Input: dimensioned drawing with shaded views. Units: mm. Origin: part minimum x, y, z. Give positions to 0.01 mm unless a question says otherwise; leave off trailing zeros. Order: outer loops, then holes, each group sorted by start corner. A loop starts at its lowest first (then second) coordinate and runs counter-clockwise, first axis right, second up.
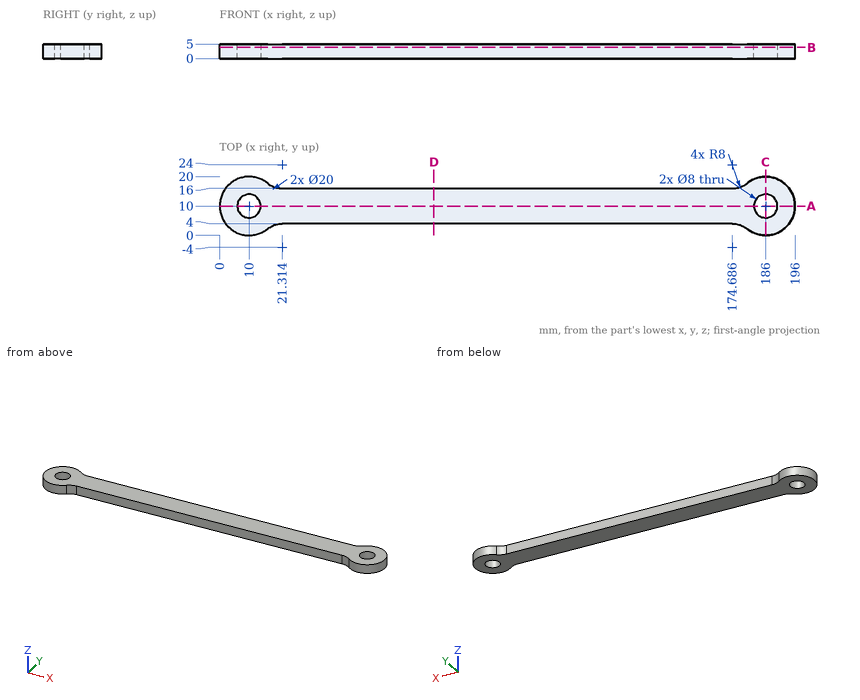
1) Section query C-C, the plane x = 186. Return the cut outline in (y, z), and give its area (3 significant figures).
Report:
outline: (0, 0) - (6, 0) - (6, 5) - (0, 5) - close; (14, 0) - (20, 0) - (20, 5) - (14, 5) - close
area: 60.0 mm2
2) Section query A-A, the plane y = 10. Return the cut outline in (x, z).
Report:
outline: (0, 0) - (6, 0) - (6, 5) - (0, 5) - close; (14, 0) - (182, 0) - (182, 5) - (14, 5) - close; (190, 0) - (196, 0) - (196, 5) - (190, 5) - close
3) Section query B-B, the plane z = 3.85. Return the cut outline in (x, y) (1 decimal).
Report:
outline: (16.3, 2.2) arc R8 cw to (21.3, 4) - (174.7, 4) arc R8 cw to (179.7, 2.2) arc R10 ccw (long way) to (179.7, 17.8) arc R8 cw to (174.7, 16) - (21.3, 16) arc R8 cw to (16.3, 17.8) arc R10 ccw (long way) to start; hole circle Ø8 at (10, 10); hole circle Ø8 at (186, 10)
4) Pin query (flat end, axial travel): pin 1 (12 mm diameter, centred on x = 90.5, y = 18, fed in from +Z); pin 2 (3 mm diameter, centred on y = 13.5, z = 2.5, fed in from +X); pin 3 (1.5 mm diameter, centred on x = 123, z = 3, fed in from +Y); pin 4 (1.5 mm diameter, centred on y = 3.5, z = 3, fed in from +X). Return the tip coordinate at first contact, or that it passes through.
Report:
pin 1: stops at z = 5
pin 2: stops at x = 195.8
pin 3: stops at y = 16
pin 4: stops at x = 194.18
5) Material intervals for L1, parallel to Y at x = 10, z = 3.65; L2, parallel to X at y = 12.5, z = 1.5; L3, parallel to X at y = 12.25, z = 2.7, sorted ascending.
Report:
L1: y = 0 to 6, 14 to 20
L2: x = 0.32 to 6.88, 13.12 to 182.88, 189.12 to 195.68
L3: x = 0.26 to 6.69, 13.31 to 182.69, 189.31 to 195.74
6) Section query D-D, the plane x = 73. Return the cut outline in (y, z), and give its area (3 significant figures).
Report:
outline: (4, 0) - (16, 0) - (16, 5) - (4, 5) - close
area: 60.0 mm2
